Job drawing, mm, ordinate dimensions from the low corner. One solid piece. A direction names the side the tool comes from. Round coordinates to 2 decimals unless told otherwise and drop trailing zeros. Write each loop counter-clockwise with the first axis right and the second up, starting at its lowest first coordinate (ties: lowest second). Pieces come first, ordered by that corner, then holes.
1) Saw through at A-A (y = 14). Write the cut outline in (x, z), plus the area to 3 significant figures.
2) Flat gauge pins, fed straight in: pin 1 (5 mm diameter, centred on x = 5.5, z = 4, fed in from -Y); pin 2 (3 mm diameter, centred on x = 10, y = 18, fed in from +Z) (3 decimals); pin 3 (5 mm diameter, centred on x = 5.5, z = 16, fed in from -Y). Where does each tip first touch, or does it go through?
3) Which spindle directions (+Z, -Z, +X, -X, +Y, -Y) get a long thin tool onto all of the face, cutting with end or side? Do the marked faces 4 and 5. Say none if no direction does.
4) Pull direction Z, two halves, no side cores. Call the marked faces 1, 2 and 3: +Z half, -Z half, draft (parallel to the pull), parting line (faces both ways), or undercut.
5) Saw through at C-C (x = 3). Write the cut outline in (y, z), plus the area to 3 significant figures.
6) Saw through at D-D (y = 24.25). Write the cut outline in (x, z).
7) Wall check: probe 1 along X at (y, z) = (25.75, 10.5); probe 2 along Z at (x, y) = (2.5, 10.5). Give the ranges that are in metal, low to high.
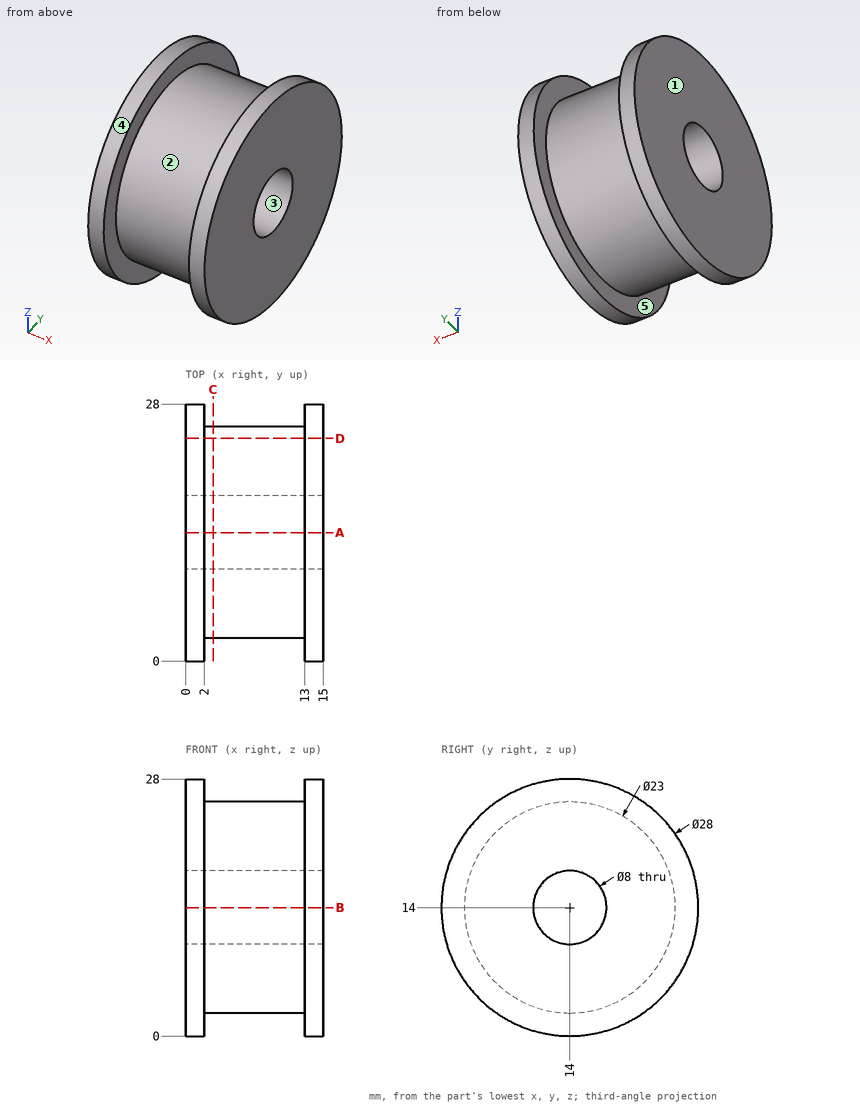
Evaluation:
1. outline: (0, 0) - (2, 0) - (2, 2.5) - (13, 2.5) - (13, 0) - (15, 0) - (15, 10) - (0, 10) - close; (0, 18) - (15, 18) - (15, 28) - (13, 28) - (13, 25.5) - (2, 25.5) - (2, 28) - (0, 28) - close
1. area: 245 mm2
2. pin 1: stops at y = 5.28
2. pin 2: stops at z = 25.225
2. pin 3: stops at y = 2.5
3. face 4: +X, -X
3. face 5: none
4. face 1: draft
4. face 2: parting line
4. face 3: undercut
5. outline: circle Ø23 at (14, 14); hole circle Ø8 at (14, 14)
5. area: 365 mm2
6. outline: (0, 4.46) - (2, 4.46) - (2, 8.79) - (13, 8.79) - (13, 4.46) - (15, 4.46) - (15, 23.54) - (13, 23.54) - (13, 19.21) - (2, 19.21) - (2, 23.54) - (0, 23.54) - close
7. probe 1: x = 0 to 2, 13 to 15
7. probe 2: z = 3.05 to 12.06, 15.94 to 24.95
